```python
from build123d import *

# Parameters (mm, degrees)
SKETCH1_W                = 96.52
SKETCH1_H                = 8.9916
MAIN_BOSS_DEPTH          = 0.8
SKETCH2_R                = 0.889
HOLES_FOR_PNP_PINS_DEPTH = 97.941215541
SKETCH3_W                = 2
SKETCH3_H                = 2.54
LOCATOR_TABS_DEPTH       = 0.2
SKETCH4_W                = 101.202450421
SKETCH4_H                = 13.068973156
SKETCH4_W_2              = 93.255989356
SKETCH4_H_2              = 5.969
CROP_DEPTH               = 97.943072319


with BuildPart() as part:
    # Sketch1 → main boss (new body)
    with BuildSketch(Plane(origin=(0, 0, 0), x_dir=(1, 0, 0), z_dir=(0, 1, 0))):
        with Locations((48.26, 4.4958)):
            Rectangle(SKETCH1_W, SKETCH1_H)
    extrude(amount=MAIN_BOSS_DEPTH)

    # Sketch2 → holes for PNP pins (cut, through all)
    with BuildSketch(Plane(origin=(0, 0, 0), x_dir=(1, 0, 0), z_dir=(0, 1, 0))):
        with Locations(Location((2.54, 3.9878, 0), (0, 0, 270))):
            Circle(SKETCH2_R)
        with Locations(Location((7.5438, 3.9878, 0), (0, 0, 270))):
            Circle(SKETCH2_R)
        with Locations(Location((12.5476, 3.9878, 0), (0, 0, 270))):
            Circle(SKETCH2_R)
        with Locations(Location((17.5514, 3.9878, 0), (0, 0, 270))):
            Circle(SKETCH2_R)
        with Locations(Location((22.5552, 3.9878, 0), (0, 0, 270))):
            Circle(SKETCH2_R)
        with Locations(Location((27.559, 3.9878, 0), (0, 0, 270))):
            Circle(SKETCH2_R)
        with Locations(Location((34.9504, 3.9878, 0), (0, 0, 270))):
            Circle(SKETCH2_R)
        with Locations(Location((39.9542, 3.9878, 0), (0, 0, 270))):
            Circle(SKETCH2_R)
        with Locations(Location((44.958, 3.9878, 0), (0, 0, 270))):
            Circle(SKETCH2_R)
        with Locations(Location((49.9618, 3.9878, 0), (0, 0, 270))):
            Circle(SKETCH2_R)
        with Locations(Location((54.9656, 3.9878, 0), (0, 0, 270))):
            Circle(SKETCH2_R)
        with Locations(Location((59.9694, 3.9878, 0), (0, 0, 270))):
            Circle(SKETCH2_R)
        with Locations(Location((67.1576, 3.9878, 0), (0, 0, 270))):
            Circle(SKETCH2_R)
        with Locations(Location((72.1614, 3.9878, 0), (0, 0, 270))):
            Circle(SKETCH2_R)
        with Locations(Location((77.1652, 3.9878, 0), (0, 0, 270))):
            Circle(SKETCH2_R)
        with Locations(Location((82.169, 3.9878, 0), (0, 0, 270))):
            Circle(SKETCH2_R)
        with Locations(Location((87.1728, 3.9878, 0), (0, 0, 270))):
            Circle(SKETCH2_R)
        with Locations(Location((92.1766, 3.9878, 0), (0, 0, 270))):
            Circle(SKETCH2_R)
    extrude(amount=HOLES_FOR_PNP_PINS_DEPTH, mode=Mode.SUBTRACT)

    # Sketch3 → locator tabs (add)
    with BuildSketch(Plane(origin=(0, 0.8, 0), x_dir=(1, 0, 0), z_dir=(0, 1, 0))):
        with Locations((7.5438, 6.7818)):
            Rectangle(SKETCH3_W, SKETCH3_H)
        with Locations((2.54, 6.7818)):
            Rectangle(SKETCH3_W, SKETCH3_H)
        with Locations((34.9504, 6.7818)):
            Rectangle(SKETCH3_W, SKETCH3_H)
        with Locations((67.1576, 6.7818)):
            Rectangle(SKETCH3_W, SKETCH3_H)
        with Locations((12.5476, 6.7818)):
            Rectangle(SKETCH3_W, SKETCH3_H)
        with Locations((17.5514, 6.7818)):
            Rectangle(SKETCH3_W, SKETCH3_H)
        with Locations((22.5552, 6.7818)):
            Rectangle(SKETCH3_W, SKETCH3_H)
        with Locations((27.559, 6.7818)):
            Rectangle(SKETCH3_W, SKETCH3_H)
        with Locations((39.9542, 6.7818)):
            Rectangle(SKETCH3_W, SKETCH3_H)
        with Locations((44.958, 6.7818)):
            Rectangle(SKETCH3_W, SKETCH3_H)
        with Locations((49.9618, 6.7818)):
            Rectangle(SKETCH3_W, SKETCH3_H)
        with Locations((54.9656, 6.7818)):
            Rectangle(SKETCH3_W, SKETCH3_H)
        with Locations((59.9694, 6.7818)):
            Rectangle(SKETCH3_W, SKETCH3_H)
        with Locations((72.1614, 6.7818)):
            Rectangle(SKETCH3_W, SKETCH3_H)
        with Locations((77.1652, 6.7818)):
            Rectangle(SKETCH3_W, SKETCH3_H)
        with Locations((82.169, 6.7818)):
            Rectangle(SKETCH3_W, SKETCH3_H)
        with Locations((87.1728, 6.7818)):
            Rectangle(SKETCH3_W, SKETCH3_H)
        with Locations((92.1766, 6.7818)):
            Rectangle(SKETCH3_W, SKETCH3_H)
    extrude(amount=LOCATOR_TABS_DEPTH)

    # Sketch4 → crop (cut, through all)
    with BuildSketch(Plane(origin=(0, 0, 0), x_dir=(1, 0, 0), z_dir=(0, 1, 0))):
        with Locations((47.986811927, 3.888963456)):
            Rectangle(SKETCH4_W, SKETCH4_H)
        with Locations((47.822628847, 4.8895)):
            Rectangle(SKETCH4_W_2, SKETCH4_H_2, mode=Mode.SUBTRACT)
    extrude(amount=CROP_DEPTH, mode=Mode.SUBTRACT)


solid = part.part
```
Check sheet for the modelled part. Datum: model origin and axes. Units: mm. Give positions to 0.01 mm unless a question says otherwise; leave off trailing zeros. Write each loop counter-clockwise with the first axis right and the second up, starting at its lowest first coordinate (ties: lowest second). Pieces come first, ordered by that corner, then holes. Notation, with made-up numbers: (63.5, 45) - (85.5, 45) arc R32 cw to (85.5, 71) - close; hole circle Ø4 at (-37, 80). An arc over 180 degrees is marked (long way). Answer as a JSON object with one key per item and string values. Group by question number.
1) Sectioned sample at C-C (x = 24.5). Record the cut outline in (y, z) (3 decimals).
2) Thickness scan on probe 1 along Y at (x, z) = (27, -4.8); probe 2 along Z at (x, y) = (12.5, 0.1) (3 decimals); probe 3 along Z at (x, y) = (83, 0.9). Record the ranges inside material, lowest first. Write a range as from..to.
3) Sectioned sample at B-B (y = 0.15). Give the number of separate pieces and of enclosed holes in the cut face, then the cut area to 3 significant figures.
4) Depth check by flat-ended pin: P1, Ø1, axis at x = 79.5, z = -6, coming from the +Y side. Enter the tip coordinate at first touch or a pass-through.
5) Sectioned sample at A-A (x = 2.54). Record the cut outline in (y, z) (3 decimals), then the cut area to 3 significant figures.
6) Release check for a two-part mould opening along X. For faces 1 (the face through (76.3, 0.4, -4.2)), 2 (the face through (77, 1, -7)) record: pulls with the +X half, pulls with the -X half, needs draft (parallel to the pull), parting line crosses it, or undercut.
Geometry results:
{
 "1": {"outline": "(0, -7.874) - (0.8, -7.874) - (0.8, -1.905) - (0, -1.905) - close"},
 "2": {"probe 1": "y = 0..0.8", "probe 2": "z = -7.874..-4.876, -3.1..-1.905", "probe 3": "z = -7.87..-5.51"},
 "3": {"separate pieces": "1", "enclosed holes": "18", "area": "512 mm^2"},
 "4": {"P1": "stops at y = 0.8"},
 "5": {"outline": "(0, -7.874) - (1, -7.874) - (1, -5.512) - (0.8, -5.512) - (0.8, -4.877) - (0, -4.877) - close; (0, -3.099) - (0.8, -3.099) - (0.8, -1.905) - (0, -1.905) - close", "area": "3.83 mm^2"},
 "6": {"face 1": "undercut", "face 2": "needs draft"}
}
